Verification items for this drawing (mm, ordinates from the low corner). Coordinates: 2 decimals unless noted, no trailing zeros. Loops run counter-clockwise (first coordinate to the right, second up) from the corner with the lowest first, then second, coordinate; pieces in that order, holes last. Notation, with made-up numbers: M -6,-30.75 L 9,-30.75 A16 cw 9,-6.75 Z; hole C 34.25,3.25 d2. An arc over 180 degrees is marked long. Return JSON: item names as keys, results as strings.
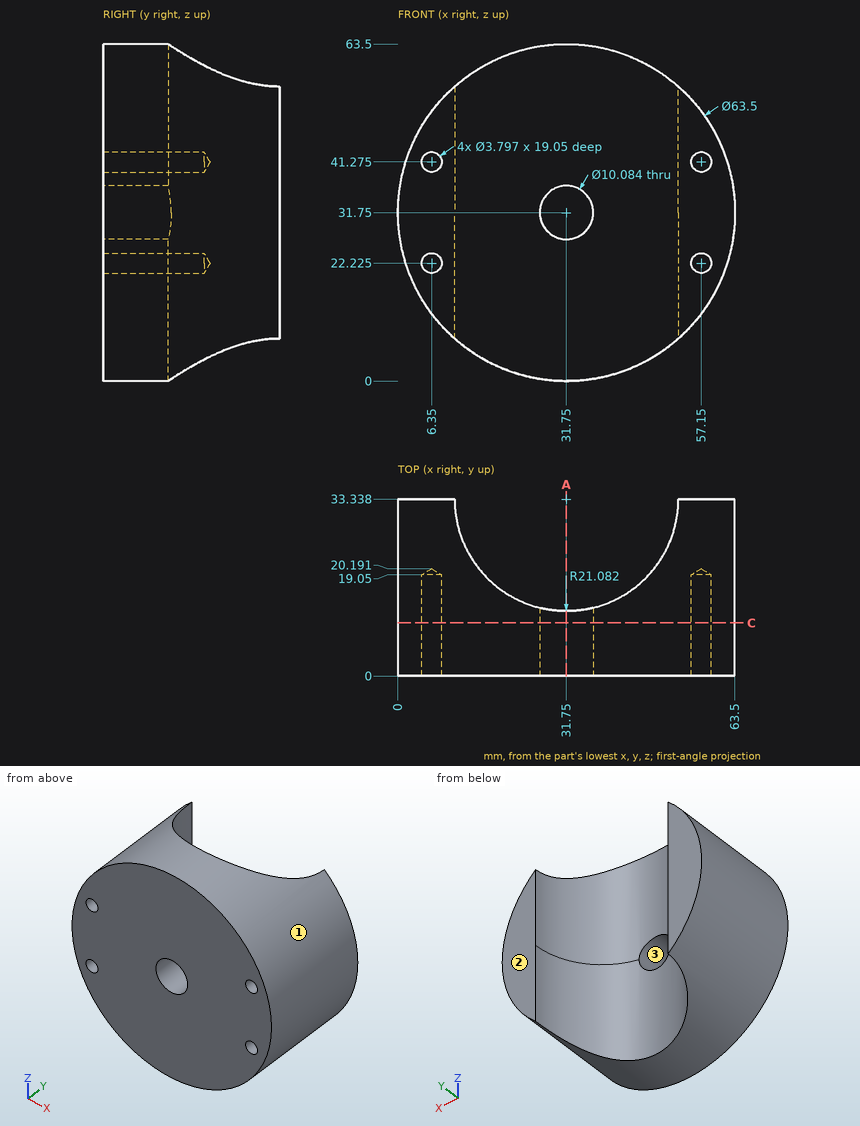
1) Section check C-C on y = 10. Count the separate pieces of the cut face and the enclosed holes in it, then the cut area to 3 significant figures.
Answers:
{"separate pieces": "1", "enclosed holes": "5", "area": "3,040 mm²"}
2) Scan lines: line 1 along Z through (x, y) = (31.75, 4); line 2 along Z through (x, y) = (6.35, 4.5) (1 decimal); line 3 along Z through (x, y) = (57, 13) (1 decimal). Record each from-to range of solid material in increasing order. Write a range as [from, to].
Answers:
{"line 1": "[0, 26.71], [36.79, 63.5]", "line 2": "[12.7, 20.3], [24.1, 39.4], [43.2, 50.8]", "line 3": "[12.5, 20.3], [24.1, 39.4], [43.2, 51]"}
3) Go/stop test with flat-tipped pins: pin 1 Ø8 at (x, y) = (17, 28) entering from +Z; pin 2 Ø4 at (y, z) = (7, 41) entering from +X; pin 3 Ø1 at (x, z) = (22.5, 9.5) entering from +Y (1 decimal); pin 4 Ø3 at (y, z) = (27.5, 56) entering from -X. Record where each tip stops, or that it passes through.
Answers:
{"pin 1": "through", "pin 2": "x = 62.66", "pin 3": "y = 14.6", "pin 4": "x = 9.6"}
4) Draft check along X on the marked faces 1, 2 and 3. Enter one of: +X half, -X half, draft (parallel to the pull), parting line (faces both ways), or undercut.
Answers:
{"face 1": "parting line", "face 2": "draft", "face 3": "undercut"}
5) Section check A-A on x = 31.75. Record the cut outline in (y, z) (1 decimal).
Answers:
{"outline": "M 0,0 L 12.3,0 L 12.3,26.7 L 0,26.7 Z; M 0,36.8 L 12.3,36.8 L 12.3,63.5 L 0,63.5 Z"}
